Can you work these out from the model? Positions are in its coordinate system, mm. Face numbers are marked on the shaded views. A direction names the side the tool comes from. Coordinates: 2 decimals unless noted, no trailing zeros. Order: outer loops, then holes, each group sorted by start corner. A loop starts at its lowest first (then second) coordinate and runs counter-clockwise, first axis right, second up. Notation, with made-up numbers: M -40,-40 L -23,-40 A19 cw -23,-19 Z; hole C 25.5,-6.5 d2. An arc over 180 degrees is marked long. Answer as CSV lines item,"result". Start each with the question number.
1. I need wall thicknesses on line 1 along Z through (x, y) = (94, 8); line 2 along Y through (x, z) = (135, -12.2). Which ranges of each line are inside material? Lowest first, please. Write a range as from..to.
2. If we section it at C-C (y = 0): Give the number of separate pieces and of enclosed holes in the cut face, plus the area to 3 significant figures.
3. If we section it at A-A (x = 75): List the corners of the cut face in (y, z) for me, plus the area to 3 significant figures.
4. If we section it at D-D (x = 114.5): List the corners of the cut face in (y, z) for me.
5. If we mould it in two halves opening along Y, with no side actions, what happens to the marked faces 3, 4 and 5? For each: released by +Y, released by -Y, zero draft, split by the parting line, or undercut.
6. If we section it at B-B (z = -4.5): List the corners of the cut face in (x, y) for me.
7. On a 3-axis mill with a long thin cutter (end or side, diameter ignored), from which of +Z, -Z, +X, -X, +Y, -Y can I reach the whole of each face in a straight line? I mean the marked faces 1 and 2. Say none if no direction works.
```python
from build123d import *

# Parameters (mm, degrees)
SKETCH1_W           = 25
SKETCH1_H           = 25
SKETCH1_W_2         = 23
SKETCH1_H_2         = 23
BOSS_EXTRUDE1_DEPTH = 150
SKETCH2_R           = 4
SKETCH2_R_2         = 5
CUT_EXTRUDE1_DEPTH  = 153.581945197


with BuildPart() as part:
    # Sketch1 → Boss-Extrude1 (new body)
    with BuildSketch(Plane(origin=(0, 0, 0), x_dir=(0, 0, -1), z_dir=(1, 0, 0))):
        Rectangle(SKETCH1_W, SKETCH1_H)
        Rectangle(SKETCH1_W_2, SKETCH1_H_2, mode=Mode.SUBTRACT)
    extrude(amount=BOSS_EXTRUDE1_DEPTH)

    # Sketch2 → Cut-Extrude1 (cut, through all)
    with BuildSketch(Plane.XY.offset(12.5)):
        with Locations((75, 0)):
            Circle(SKETCH2_R)
        with Locations((15, 0)):
            Circle(SKETCH2_R_2)
        with Locations((135, 0)):
            Circle(SKETCH2_R_2)
    extrude(amount=-CUT_EXTRUDE1_DEPTH, mode=Mode.SUBTRACT)


solid = part.part
```
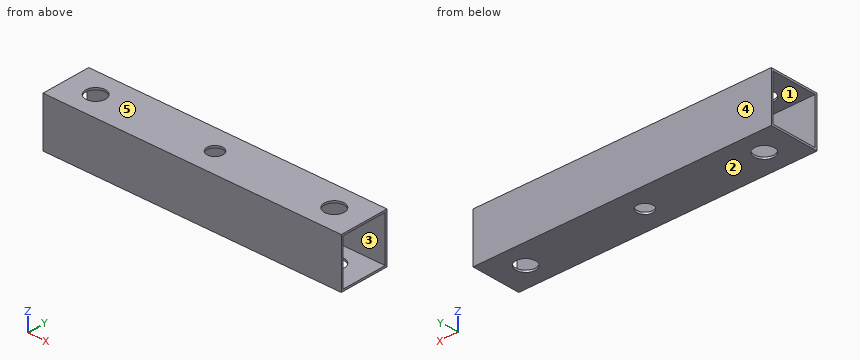
Solved:
1,line 1,"-12.5..-11.5, 11.5..12.5"
1,line 2,"-12.5..-5, 5..12.5"
2,separate pieces,"8"
2,enclosed holes,"0"
2,area,"244 mm²"
3,outline,"M -12.5,-12.5 L -4,-12.5 L -4,-11.5 L -11.5,-11.5 L -11.5,11.5 L -4,11.5 L -4,12.5 L -12.5,12.5 Z; M 4,-12.5 L 12.5,-12.5 L 12.5,12.5 L 4,12.5 L 4,11.5 L 11.5,11.5 L 11.5,-11.5 L 4,-11.5 Z"
3,area,"80.0 mm²"
4,outline,"M -12.5,-12.5 L 12.5,-12.5 L 12.5,12.5 L -12.5,12.5 Z; hole M -11.5,-11.5 L 11.5,-11.5 L 11.5,11.5 L -11.5,11.5 Z"
5,face 3,"undercut"
5,face 4,"released by +Y"
5,face 5,"zero draft"
6,outline,"M 0,-12.5 L 150,-12.5 L 150,-11.5 L 0,-11.5 Z; M 0,11.5 L 150,11.5 L 150,12.5 L 0,12.5 Z"
7,face 1,"+X, -X"
7,face 2,"-Z, +X, -X, +Y, -Y"
